```python
from build123d import *

# Parameters (mm, degrees)
SKETCH_1_W      = 55
SKETCH_1_H      = 36.8
SKETCH_1_R      = 2.1
EXTRUDE_1_DEPTH = 24


with BuildPart() as part:
    # 草图1 → 凸台-拉伸1 (new body)
    with BuildSketch(Plane.XY):
        Rectangle(SKETCH_1_W, SKETCH_1_H)
        with Locations((-20, 14.35)):
            Circle(SKETCH_1_R, mode=Mode.SUBTRACT)
        with Locations((20, 0)):
            Circle(SKETCH_1_R, mode=Mode.SUBTRACT)
        with Locations(Location((-20, -14.35, 0), (0, 0, 180))):
            Circle(SKETCH_1_R, mode=Mode.SUBTRACT)
    extrude(amount=EXTRUDE_1_DEPTH)


solid = part.part
```
Read the model definition and answer for the solid it produces. Units are mm, in the model's axes. Give positions to 0.01 mm unless a question says otherwise; leave off trailing zeros. Order: outer loops, then holes, each group sorted by start corner. A loop starts at its lowest first (then second) coordinate and runs counter-clockwise, first axis right, second up. Notation, with made-up numbers: (-12.5, 54.25) -> (16.5, 54.25) arc R17 ccw to (16.5, 87.25) -> close; hole circle Ø3 at (30, 54). An arc over 180 degrees is marked (long way). One line per item, written item: value. Start each with the question number.
(1) The part is cut by section A-A (x = -20). Determine the outline of the cut face in (y, z), and give its area (3 significant figures).
(2) Straight lines are drawn through the part: L1, parallel to Y at x = -20, z = 14; L2, parallel to Y at x = 20, z = 8.5; L3, parallel to X at y = 1, z = 22. For each, find the intervals that lie inside material, in ascending order.
(3) The part is cut by section C-C (z = 13.5). Determine the outline of the cut face in (x, y).
(4) The part is cut by section B-B (y = -14.35). Determine the outline of the cut face in (x, z), and give its area (3 significant figures).
(5) For a pull along X with two mould halves and no side action, classify faces 1 (the flat face through (-27.5, 0, 12)), 2 (the flat face through (0, 0, 24)), 3 (the cylindrical face through (-19.031, 12.487, 11.832)), 4 (the flat face through (27.5, 0, 12)) as released by +X, released by -X, zero draft, split by the parting line, or undercut.
Taken from the geometry:
1. outline: (-18.4, 0) -> (-16.45, 0) -> (-16.45, 24) -> (-18.4, 24) -> close; (-12.25, 0) -> (12.25, 0) -> (12.25, 24) -> (-12.25, 24) -> close; (16.45, 0) -> (18.4, 0) -> (18.4, 24) -> (16.45, 24) -> close
1. area: 682 mm^2
2. L1: -18.4 to -16.45, -12.25 to 12.25, 16.45 to 18.4
2. L2: -18.4 to -2.1, 2.1 to 18.4
2. L3: -27.5 to 18.15, 21.85 to 27.5
3. outline: (-27.5, -18.4) -> (27.5, -18.4) -> (27.5, 18.4) -> (-27.5, 18.4) -> close; hole circle Ø4.2 at (-20, -14.35); hole circle Ø4.2 at (-20, 14.35); hole circle Ø4.2 at (20, 0)
4. outline: (-27.5, 0) -> (-22.1, 0) -> (-22.1, 24) -> (-27.5, 24) -> close; (-17.9, 0) -> (27.5, 0) -> (27.5, 24) -> (-17.9, 24) -> close
4. area: 1,220 mm^2
5. face 1: released by -X
5. face 2: zero draft
5. face 3: undercut
5. face 4: released by +X
